Drawing for the job (mm, zero at the part's lowest x, y, z). A direction names the side the tool comes from. Round coordinates to 2 decimals unless told otherwise and drop trailing zeros. Loops run counter-clockwise (first coordinate to the right, second up) from the corner with the lowest first, then second, coordinate; pieces in that order, holes last. Notation, with made-up numbers: (-12.75, 38.5) - (40.25, 38.5) arc R25 cw to (40.25, 68.5) - close; hole circle Ø6 at (67, 48). An arc over 180 degrees is marked (long way). Put each result on its own line as item: value.
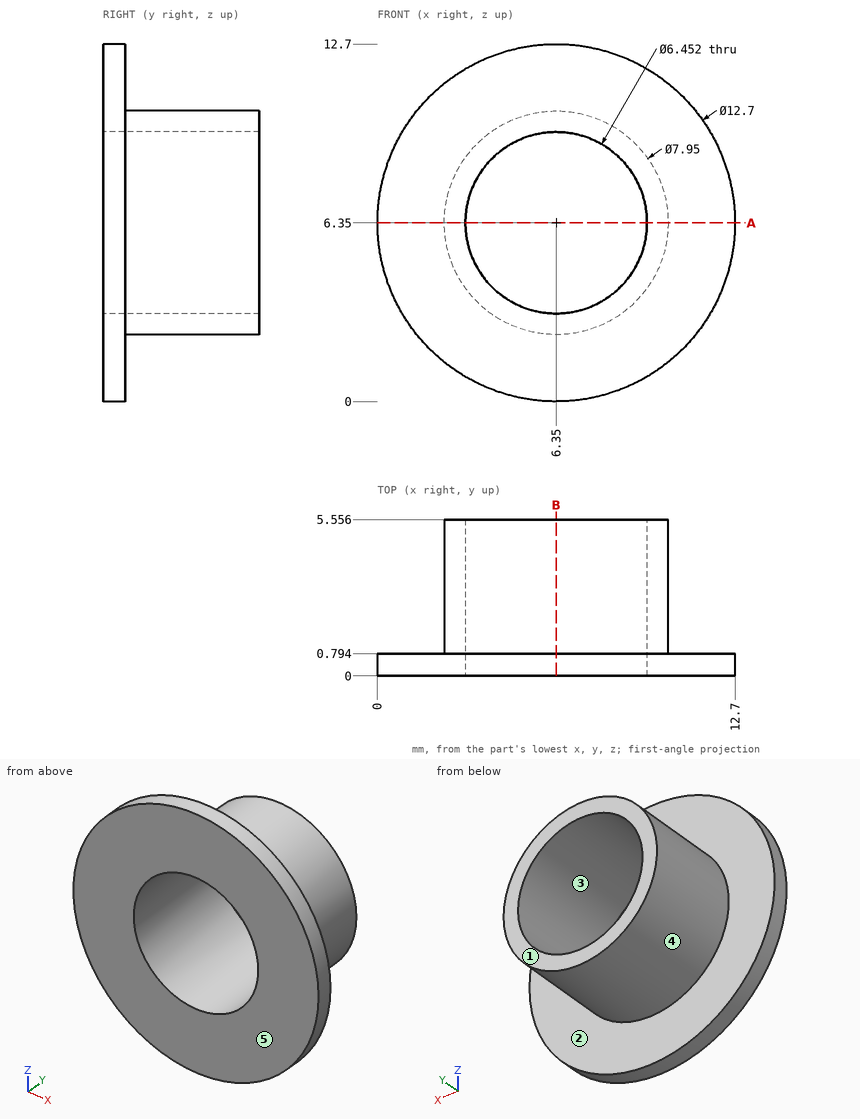
1. Probe line 1 along Z through (x, y) = (6.35, 3.65) (1 decimal); line 2 along Y through (x, z) = (6.25, 10.75). List the from-to ranges inside material, lowest first. Write a range as [from, to].
A:
line 1: z = [2.4, 3.1], [9.6, 10.3]
line 2: y = [0, 0.79]
2. Band-saw the part on A-A (z = 6.35). List the corners of the cut face in (x, y) (1 decimal).
A:
outline: (0, 0) - (3.1, 0) - (3.1, 5.6) - (2.4, 5.6) - (2.4, 0.8) - (0, 0.8) - close; (9.6, 0) - (12.7, 0) - (12.7, 0.8) - (10.3, 0.8) - (10.3, 5.6) - (9.6, 5.6) - close
3. Band-saw the part on B-B (x = 6.35). List the corners of the cut face in (y, z) (1 decimal), plus the area to 3 significant figures.
A:
outline: (0, 0) - (0.8, 0) - (0.8, 2.4) - (5.6, 2.4) - (5.6, 3.1) - (0, 3.1) - close; (0, 9.6) - (5.6, 9.6) - (5.6, 10.3) - (0.8, 10.3) - (0.8, 12.7) - (0, 12.7) - close
area: 12.1 mm²
4. Pin check, flat tips, straight feed: P1, Ø1, axis at x = 10.5, z = 7, coming from the +Y side; P2, Ø1, axis at x = 5.5, z = 6.5, coming from the +Y side; P3, Ø3, axis at y = 2.5, z = 5.5, coming from the +X side (1 decimal); P4, Ø3, axis at x = 2, y = 0.5, coming from the -Z side (1 decimal). Stop position of each tip, or through.
A:
P1: stops at y = 5.56
P2: passes through
P3: stops at x = 10.3
P4: stops at z = 0.7
5. Two-plate mould, pull along X, no slides. Class the marked faces 3, 4 and 5: pulls with the +X half, pulls with the -X half, needs draft (parallel to the pull), parting line crosses it, or undercut.
A:
face 3: undercut
face 4: parting line crosses it
face 5: needs draft
6. Tool access for the marked faces 1 and 2: list every direction of +Z, -Z, +X, -X, +Y, -Y with a clear straight run to the whole face (end or side of a thin tool).
A:
face 1: +Z, -Z, +X, -X, +Y
face 2: +Y
